from build123d import *

# Parameters (mm, degrees)
F1_DEPTH = 20
F2_R     = 5
F3_R     = 6.35
F4_DEPTH = 25
F5_R     = 3


# Not quite as in the source:
# - a feature names something its author has since deleted; it is built from what else it names


with BuildPart() as f1:
    # F0 (on Top) → F1 (new body)
    with BuildSketch(Plane.XY):
        with BuildLine():
            Line((-90.3923048454, -24.3281582892), (-90.392, -30.3281582892))
            Line((-90.392, -30.3281582892), (0, -30.3281582892))
            Line((0, -30.3281582892), (25, -30.3281582892))
            ThreePointArc((25, -30.3281582892), (-1.9589555892, -17.2068745453), (-20.9641016151, 5.9827308433))
            Line((-20.9641016151, 5.9827308433), (-31.9301010618, 24.9763990407))
            ThreePointArc((-31.9301010618, 24.9763990407), (-36.0778921244, 46.2412468008), (-23.9743052597, 64.2106960401))
            ThreePointArc((-23.9743052597, 64.2106960401), (-22.4887853878, 65.1306303747), (-20.9493389483, 65.9571611543))
            Line((-20.9493389483, 65.9571611543), (9.3615501841, 83.4571611543))
            Line((9.3615501841, 83.4571611543), (6.3615501841, 88.653313577))
            Line((6.3615501841, 88.653313577), (-49.9301010618, 56.153313577))
            Line((-49.9301010618, 56.153313577), (-56.9301010618, 68.2776692299))
            Line((-56.9301010618, 68.2776692299), (-62.1262534846, 65.2776692299))
            Line((-62.1262534846, 65.2776692299), (-53.6935750346, 50.6718417108))
            Line((-53.6935750346, 50.6718417108), (-17.8923048454, -11.3377772324))
            ThreePointArc((-17.8923048454, -11.3377772324), (-17.7483786227, -11.5778506661), (-17.6124320417, -11.8225311482))
            Line((-17.6124320417, -11.8225311482), (-10.3923048454, -24.3281582892))
            Line((-10.3923048454, -24.3281582892), (-24.8325592379, -24.3281582892))
            ThreePointArc((-24.8325592379, -24.3281582892), (-25.1124320417, -24.3327653375), (-25.3923048454, -24.3281582892))
            Line((-25.3923048454, -24.3281582892), (-90.3923048454, -24.3281582892))
        make_face()
        with BuildLine():
            ThreePointArc((-17.6124320417, -11.8225311482), (-17.7483786227, -20.0811271137), (-24.8325592379, -24.3281582892))
            Line((-24.8325592379, -24.3281582892), (-10.3923048454, -24.3281582892))
            Line((-10.3923048454, -24.3281582892), (-17.6124320417, -11.8225311482))
        make_face()
    extrude(amount=F1_DEPTH)

    # F2
    f2_edges = [f1.edges().sort_by_distance(p)[0] for p in [
        (-90.392305, -24.328158, 10),
        (-62.126253, 65.277669, 10),
        (9.36155, 83.457161, 10),
    ]]
    fillet(f2_edges, radius=F2_R)

    # F3 (on face) → F4 (cut)
    with BuildSketch(Plane.XY.offset(20)):
        with Locations((-43.719941363, 50.0970014554)):
            Circle(F3_R)
        with Locations((-9.4799492508, -22.3026443273)):
            Circle(F3_R)
    extrude(amount=-F4_DEPTH, mode=Mode.SUBTRACT)

    # F5
    f5_edges = [f1.edges().sort_by_distance(p)[0] for p in [
        (25, -30.328158, 10),
    ]]
    fillet(f5_edges, radius=F5_R)


solid = f1.part
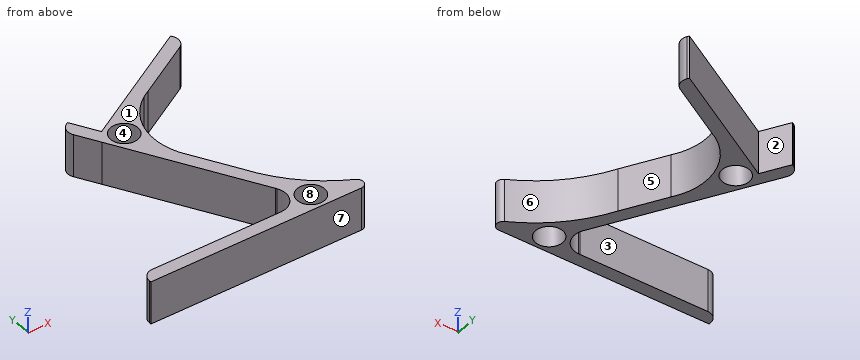
Input: part model. Units: mm. Frame: model coordinates. Face numbers are marked on the shaded views. A direction names the side the tool comes from. Round coordinates to 2 decimals unless told otherwise and drop trailing zeros. Loops run counter-clockwise (first coordinate to the right, second up) from the corner with the lowest first, then second, coordinate; pieces in that order, holes last. Notation, with made-up numbers: M 32.25,-29 L 78.25,-29 A14 cw 78.25,-6 Z; hole C -27,-25 d4. An arc over 180 degrees is marked long. Answer as CSV lines item,"result". Start each with the question number.
(1) Draft query along X for the marked faces 6, 7 and 8. Return one class per face: released by +X, released by -X, zero draft, split by the parting line, or undercut.
(2) First-contact query: pin 1 (20.5 mm diameter, centred on x = -43.72, y = 50.1, fed in from +Z); pin 2 (1 mm diameter, centred on y = -14.5, z = 7.5, fed in from -X); pin 3 (10 mm diameter, centred on x = -55.5, z = 17.5, fed in from +Y); pin 4 (1.5 mm diameter, centred on y = -1.5, z = 10.5, fed in from -X). Flat tips, straight axial feed; report the tip coordinate or a pass-through.
(3) Section D-D, the plane y = 1. Output: boundary loops of the cut face in (x, z).
(4) Reachability of the marked faces 1, 2, 3, 4 and 5 from +Z, -Z, +X, -X, +Y, -Y: full face, straight path, thin tool, end or side. Return the list, or none.
(5) Section A-A, the plane x = 2. Output: boundary loops of the cut face in (y, z).
(6) Section B-B, the plane z = 12.75. Output: boundary loops of the cut face in (x, y), plus the area to 3 significant figures.
(7) Section C-C, the plane x = -47. Output: boundary loops of the cut face in (y, z) (3 decimals).
(8) Line query: line 1 (Y direction, x = -27.5, z = 14.5); line 2 (Y direction, x = -23, z = 10.25); line 3 (Y direction, x = -79, z = 9). Output: solid intervals per line, ascending. Write a range as [from, to].
Values found:
1,face 6,"released by +X"
1,face 7,"zero draft"
1,face 8,"undercut"
2,pin 1,"stops at z = 20"
2,pin 2,"stops at x = -16.81"
2,pin 3,"stops at y = 68.28"
2,pin 4,"stops at x = -24.01"
3,outline,"M -25.02,0 L -18.17,0 L -18.17,20 L -25.02,20 Z"
4,face 1,"+Z, +X, -X, +Y, -Y"
4,face 2,"+Z, -Z, +Y"
4,face 3,"+Z, -Z, -X"
4,face 4,"+Z, -Z"
4,face 5,"+Z, -Z, +X"
5,outline,"M -30.33,0 L -20.11,0 L -20.11,20 L -30.33,20 Z; M 79.21,0 L 86.14,0 L 86.14,20 L 79.21,20 Z"
6,outline,"M -90.39,-30.33 L 8.3,-30.33 A3 ccw 9.66,-24.66 A70.06 cw -20.96,5.98 L -31.93,24.98 A28.31 cw -20.95,65.96 L 5.03,80.96 A5 ccw 6.86,87.79 L 6.36,88.65 L -49.93,56.15 L -56.93,68.28 L -57.8,67.78 A5 ccw -59.63,60.95 L -17.89,-11.34 A8.5 cw -25.39,-24.33 L -85.39,-24.33 A5 ccw -90.39,-29.33 Z; hole C -43.72,50.1 d12.7; hole C -9.48,-22.3 d12.7"
6,area,"1,670 mm²"
7,outline,"M -30.328,0 L -24.328,0 L -24.328,20 L -30.328,20 Z; M 39.078,0 L 44.66,0 L 44.66,20 L 39.078,20 Z; M 55.534,0 L 57.845,0 L 57.845,20 L 55.534,20 Z"
8,line 1,"y = [-30.33, -24.33], [5.3, 17.3], [61.45, 69.1]"
8,line 2,"y = [-30.33, -24.07], [-2.49, 9.51], [64.83, 71.7]"
8,line 3,"y = [-30.33, -24.33]"
